For this review, take the finished solid that the model builds, in its own axes (mm). Face numbers are marked on the shaded views. A direction names the side the tool comes from. Give positions to 0.01 mm unless a question says otherwise; leave off trailing zeros. Loops run counter-clockwise (first coordinate to the right, second up) from the corner with the lowest first, then second, coordinate; pieces in that order, holes last.
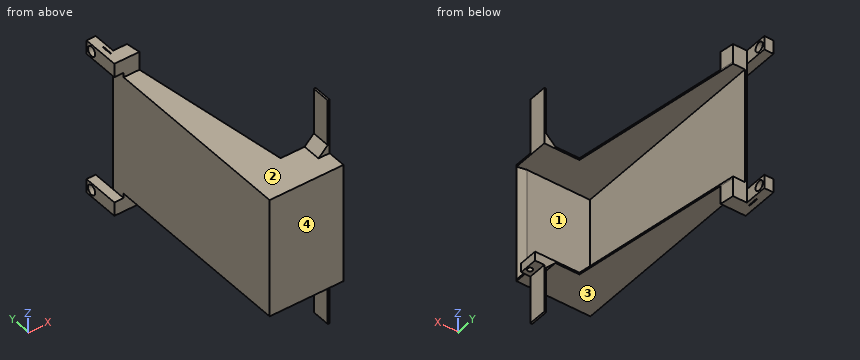
```python
from build123d import *

# Parameters (mm, degrees)
BOSS_EXTRUDE2_DEPTH = 65
CUT_EXTRUDE1_DEPTH  = 63
BOSS_EXTRUDE6_DEPTH = 20
SKETCH26_W          = 15
SKETCH26_H          = 40
BOSS_EXTRUDE7_DEPTH = 10
SKETCH27_R          = 0.5
CUT_EXTRUDE3_DEPTH  = 5
SKETCH29_R          = 5.25
CUT_EXTRUDE4_DEPTH  = 10
SKETCH30_W          = 2
SKETCH30_H          = 20
BOSS_EXTRUDE8_DEPTH = 60
CHAMFER1_SIZE       = 10
SKETCH32_W          = 10
SKETCH32_H          = 20
BOSS_EXTRUDE9_DEPTH = 10
SKETCH33_R          = 2.65
CUT_EXTRUDE5_DEPTH  = 10


with BuildPart() as part:
    # Sketch2 → Boss-Extrude2 (new, symmetric)
    with BuildSketch(Plane.XY):
        Polygon((15, 225), (0, 225), (0, 0), (80, 0), (80, 40), (42, 40), align=None)
    extrude(amount=BOSS_EXTRUDE2_DEPTH, both=True)

    # Sketch5 → Cut-Extrude1 (cut, symmetric)
    with BuildSketch(Plane.XY):
        Polygon((2, 2), (70.202041029, 2), (80, 0), (80, 40), (42, 40), (15, 225), (2, 225), align=None)
    extrude(amount=CUT_EXTRUDE1_DEPTH, both=True, mode=Mode.SUBTRACT)

    # Sketch25 → Boss-Extrude6 (add)
    with BuildSketch(Plane.XY.offset(65)):
        Polygon((17.189189189, 210), (15, 225), (0, 225), (0, 210), align=None)
    extrude(amount=BOSS_EXTRUDE6_DEPTH)

    # Sketch26 → Boss-Extrude7 (add)
    with BuildSketch(Plane.ZY):
        with Locations((77.5, 230)):
            Rectangle(SKETCH26_W, SKETCH26_H)
    extrude(amount=BOSS_EXTRUDE7_DEPTH)

    # Sketch27 → Cut-Extrude3 (cut)
    with BuildSketch(Plane.XY.offset(85)):
        with Locations((-3.905405405, 231.7)):
            Circle(SKETCH27_R)
        with Locations((-3.905405405, 233.7)):
            Circle(SKETCH27_R)
        with Locations((-3.905405405, 229.7)):
            Circle(SKETCH27_R)
        with Locations((-3.905405405, 227.7)):
            Circle(SKETCH27_R)
        with Locations((-3.905405405, 225.7)):
            Circle(SKETCH27_R)
        with Locations((-3.905405405, 223.7)):
            Circle(SKETCH27_R)
    extrude(amount=-CUT_EXTRUDE3_DEPTH, mode=Mode.SUBTRACT)

    # Sketch29 → Cut-Extrude4 (cut)
    with BuildSketch(Plane(origin=(0, 0, 0), x_dir=(0, 0, -1), z_dir=(1, 0, 0))):
        with Locations((-77.5, 242.75)):
            Circle(SKETCH29_R)
    extrude(amount=-CUT_EXTRUDE4_DEPTH, mode=Mode.SUBTRACT)

    # Sketch30 → Boss-Extrude8 (add)
    with BuildSketch(Plane.XY.offset(65)):
        with Locations((79, 30)):
            Rectangle(SKETCH30_W, SKETCH30_H)
    extrude(amount=BOSS_EXTRUDE8_DEPTH)

    # Chamfer1
    chamfer1_edges = [part.edges().sort_by_distance(p)[0] for p in [
        (78, 30, 65),
    ]]
    chamfer(chamfer1_edges, length=CHAMFER1_SIZE)

    # Mirror3: part across plane


with BuildPart() as part_1:
    add(part.part)
    add(part.part.mirror(Plane(origin=(0, 0, 0), x_dir=(1, 0, 0), z_dir=(0, 0, -1))))

    # Sketch32 → Boss-Extrude9 (add)
    with BuildSketch(Plane(origin=(80, 0, 0), x_dir=(0, 0, -1), z_dir=(1, 0, 0))):
        with Locations((68, 30)):
            Rectangle(SKETCH32_W, SKETCH32_H)
    extrude(amount=BOSS_EXTRUDE9_DEPTH)

    # Sketch33 → Cut-Extrude5 (cut)
    with BuildSketch(Plane.XY.offset(-63)):
        with Locations((86, 27.5)):
            Circle(SKETCH33_R)
    extrude(amount=-CUT_EXTRUDE5_DEPTH, mode=Mode.SUBTRACT)


solid = part_1.part
```
Item 1: Tool access review of the marked faces 1, 2, 3 and 4: name each direction out of +Z, -Z, +X, -X, +Y, -Y from which nothing blocks a thin tool from reaching the whole face with its end or side.
Answer:
face 1: +X, +Y
face 2: +Z, -X, -Y
face 3: -Z, -X, -Y
face 4: +Z, -Z, +X, -X, -Y
Item 2: Take a section at B-B on y = 77. Give the boundary of the cut face in (x, z).
Answer:
outline: (0, -65) - (36.6, -65) - (36.6, -63) - (2, -63) - (2, 63) - (36.6, 63) - (36.6, 65) - (0, 65) - close
Item 3: For L1, parallel to Z at x = 14, y = 22; L2, parallel to Y at x = 86, z = -66.25; L3, parallel to X at y = 233.7, z = -82, list the stretches that pass through material, from the lowest coordinate up.
Answer:
L1: z = -65 to -63, 63 to 65
L2: y = 20 to 24.85, 30.15 to 40
L3: x = -10 to -4.41, -3.41 to 0
Item 4: Clearance check with flat-ended pins moving along their axes: pin 1 Ø0.8 at (x, y) = (-3.5, 232) entering from +Z; pin 2 Ø7.5 at (y, z) = (242, -80) entering from +X; pin 3 Ø6 at (x, z) = (69, -5) entering from +Y; pin 4 Ø5 at (x, y) = (86, 27.5) entering from -Z. State where each tip first meets the part, or that it passes through.
Answer:
pin 1: stops at z = 85
pin 2: stops at x = 0
pin 3: stops at y = 2
pin 4: passes through
Item 5: Take a section at C-C on z = -23.5. Give the boundary of the cut face in (x, y), and give its area (3 significant figures).
Answer:
outline: (0, 0) - (80, 0) - (70.2, 2) - (2, 2) - (2, 225) - (0, 225) - close
area: 596 mm2
Item 6: Take a section at D-D on y = 103. Give the boundary of the cut face in (x, z).
Answer:
outline: (0, -65) - (32.81, -65) - (32.81, -63) - (2, -63) - (2, 63) - (32.81, 63) - (32.81, 65) - (0, 65) - close
Item 7: Take a section at A-A on y = 242.75. Give the boundary of the cut face in (x, z).
Answer:
outline: (-10, -85) - (0, -85) - (0, -82.75) - (-10, -82.75) - close; (-10, -72.25) - (0, -72.25) - (0, -70) - (-10, -70) - close; (-10, 70) - (0, 70) - (0, 72.25) - (-10, 72.25) - close; (-10, 82.75) - (0, 82.75) - (0, 85) - (-10, 85) - close
